Here's how the part is built. I have some questions about the finished solid (model axes, mm). A direction names the side the tool comes from. Give positions to 0.01 mm unless a question says otherwise; leave off trailing zeros. Write each loop counter-clockwise with the first axis right and the second up, starting at its lowest first coordinate (ties: lowest second). Pieces come first, ordered by that corner, then holes. Notation, with made-up numbers: (-30.75, 84) - (10.25, 84) arc R19 cw to (10.25, 100) - close; hole circle Ø2 at (38, 24). An arc over 180 degrees is marked (long way). Write each question's results on one line, items separated by ' | '. Start each with the question number.
Item 1: Please list where these lines run through material, in increasing order: line 1 along Y through (x, z) = (0, -1.55) (3 decimals); line 2 along X through (y, z) = (10.5, -2.65); line 3 along X through (y, z) = (-3, -2.75).
Item 2: Suppose I cut it at C-C on z = -1.7. List the corners of the cut face in (x, y) for me (3 decimals).
Item 3: Will these pins go through, and if not, where does the flat tip stop? P1, Ø0.9, axis at x = -8.5, z = -1, coming from the +Y side; P2, Ø1, axis at y = 13.5, z = -2, coming from the -X side; P3, Ø4, axis at x = 15, y = 20.5, coming from the +Z side; P4, Ø0.9, axis at y = -2.5, z = -2, coming from the -X side.
Item 4: Which directions (+Z, -Z, +X, -X, +Y, -Y) give clear straight access to the entire face, cutting with the end or side of a thin tool? Please do faces 1 (the flat face through (18, 0, 0)), 2 (the flat face through (0, -17.5, -1)).
Item 5: Suppose I cut it at A-A on x = 0. List the corners of the cut face in (y, z) for me (3 decimals), then the cut area to 3 significant figures.
Item 6: Suppose I cut it at B-B on y = 0. List the corners of the cut face in (x, z) for me, then the cut area to 3 significant figures.
Item 7: Suppose I cut it at D-D on x = -11.5. List the corners of the cut face in (y, z) for me.
Autodesk Inventor part; units mm, degrees
ref_plane "YZ Plane" through (0, 0, 0) normal (1, 0, 0) x (0, 1, 0)
ref_plane "XZ Plane" through (0, 0, 0) normal (0, 1, 0) x (-1, 0, 0)
ref_plane "XY Plane" through (0, 0, 0) normal (0, 0, 1) x (1, 0, 0)
sketch "スケッチ1" plane through (0, 0, 0) normal (0, 0, 1) x (1, 0, 0)
  circle A0 centre (0, 0) radius 27.25
  line L0 (17.5, 17.5) -> (-17.5, 17.5)
  line L1 (-17.5, 17.5) -> (-17.5, -17.5)
  line L2 (-17.5, -17.5) -> (17.5, -17.5)
  line L3 (17.5, -17.5) -> (17.5, 17.5)
  line L4 (17.5, 17.5) -> (-17.5, -17.5) construction
  line L5 (-17.5, 17.5) -> (17.5, -17.5) construction
  line L6 (1, 17.5) -> (-1, 17.5)
  line L7 (-1, -17.5) -> (1, -17.5)
  dimension "d0" = 54.5
  dimension "d6" = 35
  dimension "d107" = 2
  dimension "d108" = 35
extrude "押し出し1" add sketch "スケッチ1" against normal blind 3
sketch "スケッチ8" plane through (0, 0, 0) normal (0, 0, 1) x (1, 0, 0)
  circle A0 centre (0, 0) radius 27.25
  circle A1 centre (0, 0) radius 22.375
  line L0 (0, 30.4962) -> (0, -31.0616)
  point P0 (0, 0)
  point P1 (0, 22.375)
  point P2 (0, -22.375)
  dimension "d111" = 44.75
  dimension "d112" = 54.5
hole "穴5" at (0, 22.375, 0) at (0, -22.375, 0) direction (0, 0, -1) diameter 4.5 end through all
properties part number "Part3_A_Y" material "鋼、軟鋼"
Checked values:
1) line 1: y = -27.25 to -24.625, -20.125 to -17.5, 17.5 to 20.125, 24.625 to 27.25 | line 2: x = -25.15 to -17.5, 17.5 to 25.15 | line 3: x = -27.08 to -17.5, 17.5 to 27.08
2) outline: circle Ø54.5 at (0, 0); hole (-17.5, -17.5) - (17.5, -17.5) - (17.5, 17.5) - (-17.5, 17.5) - close; hole circle Ø4.5 at (0, -22.375); hole circle Ø4.5 at (0, 22.375)
3) P1: stops at y = 26.03 | P2: stops at x = -23.95 | P3: stops at z = 0 | P4: stops at x = -27.17
4) face 1: +Z, +X, -X, +Y, -Y | face 2: +Z, -Z
5) outline: (-27.25, -3) - (-24.625, -3) - (-24.625, 0) - (-27.25, 0) - close; (-20.125, -3) - (-17.5, -3) - (-17.5, 0) - (-20.125, 0) - close; (17.5, -3) - (20.125, -3) - (20.125, 0) - (17.5, 0) - close; (24.625, -3) - (27.25, -3) - (27.25, 0) - (24.625, 0) - close | area: 31.5 mm^2
6) outline: (-27.25, -3) - (-17.5, -3) - (-17.5, 0) - (-27.25, 0) - close; (17.5, -3) - (27.25, -3) - (27.25, 0) - (17.5, 0) - close | area: 58.5 mm^2
7) outline: (-24.7, -3) - (-17.5, -3) - (-17.5, 0) - (-24.7, 0) - close; (17.5, -3) - (24.7, -3) - (24.7, 0) - (17.5, 0) - close
